from build123d import *

# Parameters (mm, degrees)
BOSS_EXTRUDE1_DEPTH = 8
SKETCH6_R           = 1.5
CUT_EXTRUDE2_DEPTH  = 50


with BuildPart() as part:
    # Sketch1 → Boss-Extrude1 (new body)
    with BuildSketch(Plane(origin=(0, 0, 0), x_dir=(0, 0, -1), z_dir=(1, 0, 0))):
        Polygon((-25, 0), (235, 0), (235, 37.995251441), (192.301615505, 50), (17.698384495, 50), (-25, 37.995251441), align=None)
    extrude(amount=BOSS_EXTRUDE1_DEPTH)

    # Sketch6 → Cut-Extrude2 (cut)
    with BuildSketch(Plane.XZ):
        with Locations(Location((4, -26.25, 0), (0, 0, 270))):
            Circle(SKETCH6_R)
        with Locations(Location((4, -78.75, 0), (0, 0, 270))):
            Circle(SKETCH6_R)
        with Locations(Location((4, -131.25, 0), (0, 0, 270))):
            Circle(SKETCH6_R)
        with Locations(Location((4, -183.75, 0), (0, 0, 270))):
            Circle(SKETCH6_R)
    extrude(amount=-CUT_EXTRUDE2_DEPTH, mode=Mode.SUBTRACT)


solid = part.part
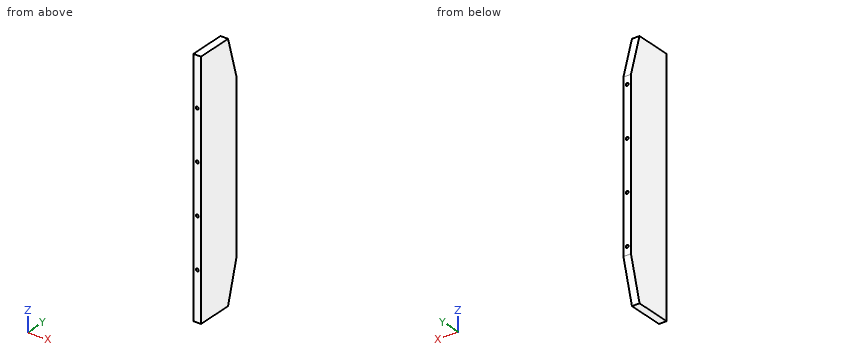
The listing builds one solid part. Answer for the finished solid, in the listing's coordinates (mm). Coordinates: 2 decimals unless noted, no trailing zeros. Order: outer loops, then holes, each group sorted by start corner. A loop starts at its lowest first (then second) coordinate and runs counter-clockwise, first axis right, second up. Notation, with made-up numbers: (-3, 42.25) -> (36, 42.25) arc R13 ccw to (36, 47.25) -> close; hole circle Ø3 at (24.25, 67.25). An arc over 180 degrees is marked (long way). Answer in a Markdown table with one row per item. Add a question column.
Item 1: Find the intervals of material crossed by L1, parallel to X at y = 35, z = -26; L2, parallel to X at y = 23.5, z = -27.5; L3, parallel to Y at x = 3.5, z = -7.5, in increasing order. Write a range as from..to.
Item 2: Find section A-A (y = 42.5). Write down the section's boundary in (x, z).
Item 3: Each of these flat-tipped pins is pushed along its axis until it touches: P1, Ø1, axis at x = 6, z = -22, coming from the -Y side; P2, Ø1.8, axis at x = 4, z = -26.25, coming from the -Y side; P3, Ø2, axis at x = 1, z = -8, coming from the +Y side. Where does it stop, or does it pass through?
Result set:
| question | item | result |
|---|---|---|
| 1 | L1 | x = 0..2.52, 5.48..8 |
| 1 | L2 | x = 0..3.17, 4.83..8 |
| 1 | L3 | y = 0..47.13 |
| 2 | outline | (0, -218.98) -> (8, -218.98) -> (8, 8.98) -> (0, 8.98) -> close; hole circle Ø3 at (4, -183.75); hole circle Ø3 at (4, -131.25); hole circle Ø3 at (4, -78.75); hole circle Ø3 at (4, -26.25) |
| 3 | P1 | stops at y = 0 |
| 3 | P2 | passes through |
| 3 | P3 | stops at y = 47.55 |
